Work out the finished part from the listing and answer in its coordinate system (mm). A direction names the side the tool comes from. Round coordinates to 2 decimals unless told otherwise and drop trailing zeros. Loops run counter-clockwise (first coordinate to the right, second up) from the corner with the lowest first, then second, coordinate; pieces in that order, holes last.
```python
from build123d import *

# Parameters (mm, degrees)
F1_DEPTH = 10
F3_DEPTH = 10
F5_DEPTH = 10
F6_W     = 20
F6_H     = 6
F6_W_2   = 6
F6_H_2   = 30
F6_H_3   = 20
F7_DEPTH = 40
F8_W     = 30
F8_H     = 5
F8_W_2   = 20
F9_DEPTH = 50.001


# Not quite as in the source:
# - a feature names something its author has since deleted; it is built from what else it names


with BuildPart() as f1:
    # F0 (on Top) → F1 (new body)
    with BuildSketch(Plane.XY):
        with BuildLine():
            Line((0, -50), (0, 0))
            Line((0, 0), (-50, 0))
            Line((-50, 0), (-50, -40))
            ThreePointArc((-50, -40), (-47.0710678119, -47.0710678119), (-40, -50))
            Line((-40, -50), (0, -50))
        make_face()
    extrude(amount=F1_DEPTH)

    # F2 (on Right) → F3 (join)
    with BuildSketch(Plane.YZ):
        with BuildLine():
            Line((-50, 10), (0, 10))
            Line((0, 10), (0, 50))
            Line((0, 50), (-40, 50))
            ThreePointArc((-40, 50), (-47.0710678119, 47.0710678119), (-50, 40))
            Line((-50, 40), (-50, 10))
        make_face()
    extrude(amount=-F3_DEPTH)

    # F4 (on Front) → F5 (join)
    with BuildSketch(Plane.XZ):
        with BuildLine():
            Line((-50, 10), (-10, 10))
            Line((-10, 10), (-10, 50))
            Line((-10, 50), (-40, 50))
            ThreePointArc((-40, 50), (-47.0710678119, 47.0710678119), (-50, 40))
            Line((-50, 40), (-50, 10))
        make_face()
    extrude(amount=F5_DEPTH)

    # F6 (on face) → F7 (cut)
    with BuildSketch(Plane.XZ.offset(50)):
        Polygon((-15, 2), (-10, 2), (-10, 8), (-40, 8), (-40, 2), align=None)
        with Locations((-50, 5)):
            Rectangle(F6_W, F6_H)
        with Locations((-5, 25)):
            Rectangle(F6_W_2, F6_H_2)
        with Locations((-5, 50)):
            Rectangle(F6_W_2, F6_H_3)
    extrude(amount=-F7_DEPTH, mode=Mode.SUBTRACT)

    # F8 (on face) → F9 (cut, through all)
    with BuildSketch(Plane.XY.offset(50)):
        with Locations((-25, -5)):
            Rectangle(F8_W, F8_H)
        with Locations((-50, -5)):
            Rectangle(F8_W_2, F8_H)
    extrude(amount=-F9_DEPTH, mode=Mode.SUBTRACT)


solid = f1.part
```
1. Determine the mould class of faces 1 (the face through (-5, -10, 30)), 2 (the face through (-30, -30, 2)), 3 (the face through (-10, -5, 25)) for opening direction Y: +Y half, -Y half, draft (parallel to the pull), parting line (faces both ways), or undercut.
Answer key:
face 1: -Y half
face 2: draft
face 3: undercut
2. Find section B-B (z = 6.5). Write down the section's boundary in (x, y), then the cut area to 3 significant figures.
Answer key:
outline: (-50, -10) - (-10, -10) - (-10, -50) - (0, -50) - (0, 0) - (-50, 0) - (-50, -2.5) - (-10, -2.5) - (-10, -7.5) - (-50, -7.5) - close
area: 700 mm2
3. Find section C-C (x = -3.5). Write down the section's boundary in (y, z).
Answer key:
outline: (-50, 0) - (0, 0) - (0, 50) - (-10, 50) - (-10, 10) - (-50, 10) - close
4. Find section D-D (y = -13). Write down the section's boundary in (x, z).
Answer key:
outline: (-50, 0) - (0, 0) - (0, 50) - (-2, 50) - (-2, 10) - (-8, 10) - (-8, 50) - (-10, 50) - (-10, 10) - (-50, 10) - (-50, 8) - (-10, 8) - (-10, 2) - (-50, 2) - close
5. Which of the six approach directions +Z, -Z, +X, -X, +Y, -Y give full straight-line access (tool end or side, diameter ignored) to faces 4 (the face through (-30, -2.5, 25)), 5 (the face through (-10, -30, 30)), 6 (the face through (-30, -30, 8))?
Answer key:
face 4: +Z, -Z, -X
face 5: +Z, -X, -Y
face 6: -X, -Y
6. Consider probe 1 along Y at (x, z) = (-45.5, 22); probe 2 along X at (y, z) = (-47.5, 26.5); probe 3 along Z at (x, y) = (-25.5, -29.5). Determine where each line is inside the solid, lowest interval first.
Answer key:
probe 1: y = -10 to -7.5, -2.5 to 0
probe 2: x = -10 to -8, -2 to 0
probe 3: z = 0 to 2, 8 to 10
7. Find section A-A (x = -20). Write down the section's boundary in (y, z), then the cut area to 3 significant figures.
Answer key:
outline: (-50, 0) - (-7.5, 0) - (-7.5, 50) - (-10, 50) - (-10, 10) - (-50, 10) - (-50, 8) - (-10, 8) - (-10, 2) - (-50, 2) - close; (-2.5, 0) - (0, 0) - (0, 50) - (-2.5, 50) - close
area: 410 mm2
8. Given pin 1 (12 mm diameter, centred on y = -21.5, z = 25.5, fed in from -X); pin 2 (6.5 mm diameter, centred on x = -4, y = -32, fed in from +Z); pin 3 (1.8 mm diameter, centred on x = -4, z = 26.5, fed in from -Y); pin 4 (1.5 mm diameter, centred on x = -37, y = -37.5, fed in from +Z), each flat-ended and moving along its own axis, determine where each tip first touches the part or whether it passes through.
Answer key:
pin 1: stops at x = -10
pin 2: stops at z = 50
pin 3: stops at y = -10
pin 4: stops at z = 10
